from build123d import *

# Parameters (mm, degrees)
BOSS_EXTRUDE1_DEPTH = 34
BOSS_EXTRUDE4_START = -34
SKETCH2_R           = 1.35
BOSS_EXTRUDE4_DEPTH = 3
BOSS_EXTRUDE5_START = 3
SKETCH3_R           = 1.35
BOSS_EXTRUDE5_DEPTH = 3
CUT_EXTRUDE1_REACH  = 149.269
SKETCH4_W           = 50
SKETCH4_H           = 5
SKETCH4_H_2         = 10
CUT_EXTRUDE3_REACH  = 122.462
SKETCH5_W           = 5
SKETCH5_H           = 25


with BuildPart() as part:
    # Sketch1 → Boss-Extrude1 (new body)
    with BuildSketch(Plane.XY):
        Polygon((-115.55, 0), (0, 0), (0, 3), (-114.069788366, 3), (-136.169180916, 31.825294631), (-138.55, 30), align=None)
    extrude(amount=BOSS_EXTRUDE1_DEPTH)

    # Sketch2 → Boss-Extrude4 (add)
    # profile 1 of 3: a face of its own
    with BuildSketch(Plane.XY.offset(34).offset(BOSS_EXTRUDE4_START)):
        Polygon((0, 3), (-114.069788366, 3), (-136.169180916, 31.825294631), (-138.55, 30), (-115.55, 0), (0, 0), align=None)
    # profile 2 of 3: a face of its own
    with BuildSketch(Plane.XY.offset(34).offset(BOSS_EXTRUDE4_START)):
        Polygon((-34.075, 36.51210805), (-34.075, 3), (0, 3), (0, 8.6), (-28.475, 8.6), (-28.475, 36.51210805), align=None)
        with Locations((-25.975, 5.8)):
            Circle(SKETCH2_R, mode=Mode.SUBTRACT)
        with Locations((-3.975, 5.8)):
            Circle(SKETCH2_R, mode=Mode.SUBTRACT)
        with Locations((-31.275, 12.1)):
            Circle(SKETCH2_R, mode=Mode.SUBTRACT)
        with Locations((-31.275, 34.1)):
            Circle(SKETCH2_R, mode=Mode.SUBTRACT)
    # profile 3 of 3: a face of its own
    with BuildSketch(Plane.XY.offset(34).offset(BOSS_EXTRUDE4_START)):
        Polygon((-104.069788366, 3), (-114.069788366, 3), (-136.169180916, 31.825294631), (-138.55, 30), (-115.55, 0), (0, 0), (0, 3), (-34.075, 3), (-100.504119084, 3), align=None)
    extrude(amount=-BOSS_EXTRUDE4_DEPTH)

    # Sketch3 → Boss-Extrude5 (add)
    with BuildSketch(Plane.XY.offset(34).offset(BOSS_EXTRUDE5_START)):
        Polygon((0, 0), (0, 3), (0, 8.6), (-28.475, 8.6), (-28.475, 36.51210805), (-34.075, 36.51210805), (-34.075, 3), (-114.069788366, 3), (-136.169180916, 31.825294631), (-138.55, 30), (-115.55, 0), align=None)
        with Locations((-31.275, 34.1)):
            Circle(SKETCH3_R, mode=Mode.SUBTRACT)
        with Locations((-31.275, 12.1)):
            Circle(SKETCH3_R, mode=Mode.SUBTRACT)
        with Locations((-25.975, 5.8)):
            Circle(SKETCH3_R, mode=Mode.SUBTRACT)
        with Locations((-3.975, 5.8)):
            Circle(SKETCH3_R, mode=Mode.SUBTRACT)
    extrude(amount=-BOSS_EXTRUDE5_DEPTH)

    # Sketch4 → Cut-Extrude1 (cut, up to next)
    with BuildSketch(Plane(origin=(0, 3, 0), x_dir=(1, 0, 0), z_dir=(0, 1, 0)), mode=Mode.PRIVATE) as cut_extrude1_sk1:
        with Locations((-79.069788366, -4.5)):
            Rectangle(SKETCH4_W, SKETCH4_H)
    cut_extrude1_tool1 = extrude(cut_extrude1_sk1.sketch, amount=-CUT_EXTRUDE1_REACH, mode=Mode.PRIVATE) & part.part
    # Sketch4 → Cut-Extrude1 (cut, up to next)
    with BuildSketch(Plane(origin=(0, 3, 0), x_dir=(1, 0, 0), z_dir=(0, 1, 0)), mode=Mode.PRIVATE) as cut_extrude1_sk2:
        with Locations((-79.069788366, -29.5)):
            Rectangle(SKETCH4_W, SKETCH4_H)
    cut_extrude1_tool2 = extrude(cut_extrude1_sk2.sketch, amount=-CUT_EXTRUDE1_REACH, mode=Mode.PRIVATE) & part.part
    # Sketch4 → Cut-Extrude1 (cut, up to next)
    with BuildSketch(Plane(origin=(0, 3, 0), x_dir=(1, 0, 0), z_dir=(0, 1, 0)), mode=Mode.PRIVATE) as cut_extrude1_sk3:
        with Locations((-79.069788366, -17)):
            Rectangle(SKETCH4_W, SKETCH4_H_2)
    cut_extrude1_tool3 = extrude(cut_extrude1_sk3.sketch, amount=-CUT_EXTRUDE1_REACH, mode=Mode.PRIVATE) & part.part
    add(cut_extrude1_tool1.solids().sort_by_distance((-79.069788, 3, 4.5))[0], mode=Mode.SUBTRACT)
    add(cut_extrude1_tool2.solids().sort_by_distance((-79.069788, 3, 29.5))[0], mode=Mode.SUBTRACT)
    add(cut_extrude1_tool3.solids().sort_by_distance((-79.069788, 3, 17))[0], mode=Mode.SUBTRACT)

    # Sketch5 → Cut-Extrude3 (cut, up to next)
    with BuildSketch(Plane(origin=(-70.393848516, -53.968617195, 0), x_dir=(0, 0, -1), z_dir=(0.7936063612919156, 0.6084315436571361, 0)), mode=Mode.PRIVATE) as cut_extrude3_sk1:
        with Locations((-19.5, 90.606381212)):
            Rectangle(SKETCH5_W, SKETCH5_H)
    cut_extrude3_tool1 = extrude(cut_extrude3_sk1.sketch, amount=-CUT_EXTRUDE3_REACH, mode=Mode.PRIVATE) & part.part
    # Sketch5 → Cut-Extrude3 (cut, up to next)
    with BuildSketch(Plane(origin=(-70.393848516, -53.968617195, 0), x_dir=(0, 0, -1), z_dir=(0.7936063612919156, 0.6084315436571361, 0)), mode=Mode.PRIVATE) as cut_extrude3_sk2:
        with Locations((-14.5, 90.606381212)):
            Rectangle(SKETCH5_W, SKETCH5_H)
    cut_extrude3_tool2 = extrude(cut_extrude3_sk2.sketch, amount=-CUT_EXTRUDE3_REACH, mode=Mode.PRIVATE) & part.part
    # Sketch5 → Cut-Extrude3 (cut, up to next)
    with BuildSketch(Plane(origin=(-70.393848516, -53.968617195, 0), x_dir=(0, 0, -1), z_dir=(0.7936063612919156, 0.6084315436571361, 0)), mode=Mode.PRIVATE) as cut_extrude3_sk3:
        with Locations((-4.5, 90.606381212)):
            Rectangle(SKETCH5_W, SKETCH5_H)
    cut_extrude3_tool3 = extrude(cut_extrude3_sk3.sketch, amount=-CUT_EXTRUDE3_REACH, mode=Mode.PRIVATE) & part.part
    # Sketch5 → Cut-Extrude3 (cut, up to next)
    with BuildSketch(Plane(origin=(-70.393848516, -53.968617195, 0), x_dir=(0, 0, -1), z_dir=(0.7936063612919156, 0.6084315436571361, 0)), mode=Mode.PRIVATE) as cut_extrude3_sk4:
        with Locations((-29.5, 90.606381212)):
            Rectangle(SKETCH5_W, SKETCH5_H)
    cut_extrude3_tool4 = extrude(cut_extrude3_sk4.sketch, amount=-CUT_EXTRUDE3_REACH, mode=Mode.PRIVATE) & part.part
    add(cut_extrude3_tool1.solids().sort_by_distance((-125.521629, 17.937183, 19.5))[0], mode=Mode.SUBTRACT)
    add(cut_extrude3_tool2.solids().sort_by_distance((-125.521629, 17.937183, 14.5))[0], mode=Mode.SUBTRACT)
    add(cut_extrude3_tool3.solids().sort_by_distance((-125.521629, 17.937183, 4.5))[0], mode=Mode.SUBTRACT)
    add(cut_extrude3_tool4.solids().sort_by_distance((-125.521629, 17.937183, 29.5))[0], mode=Mode.SUBTRACT)


solid = part.part
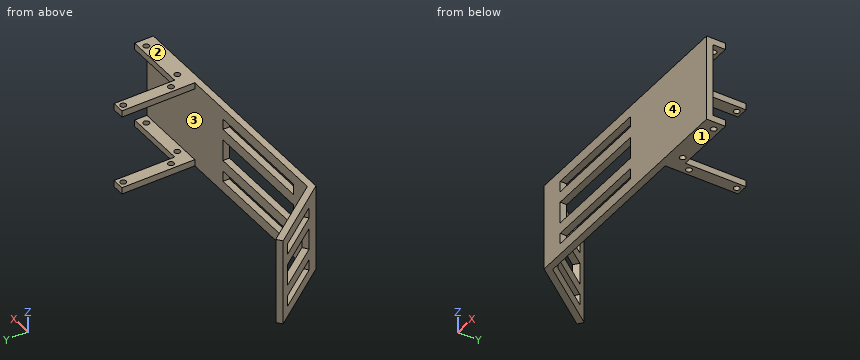
Read the model definition and answer for the solid it produces. Units are mm, in the model's axes. Face numbers are marked on the shaded views. Coordinates: 2 decimals unless noted, no trailing zeros. Loops run counter-clockwise (first coordinate to the right, second up) from the corner with the lowest first, then second, coordinate; pieces in that order, holes last. Notation, with made-up numbers: (-29.75, 49) -> (24.25, 49) arc R27 ccw to (24.25, 79) -> close; hole circle Ø9 at (14.5, 79). An arc over 180 degrees is marked (long way). Write item = value, one per line. Start each with the question number.
1) The part is cut by section D-D, the plane y = 12.1. State how many separate pieces and enclosed holes the cut face has, plus the area to 3 significant figures.
2) The mould has two halves that part along Z. Classify the marked faces 1, 2, 3 and 4: pulls with the +Z half, pulls with the -Z half, needs draft (parallel to the pull), parting line crosses it, or undercut.
3) The part is cut by section C-C, the plane x = -64.5. Determine the outline of the cut face in (y, z), plus the area to 3 significant figures.
4) The part is cut by section B-B, the plane z = 29. Determine the outline of the cut face in (x, y), plus the area to 3 significant figures.
5) Given P1, Ø1.5, axis at y = 27.5, z = 11.5, coming from the +X side; P2, Ø1.6, axis at x = -31.275, y = 12.1, coming from the +Z side; P3, Ø10, axis at y = 32.5, z = 9.5, coming from the +X side; P4, Ø2.5, axis at y = 17.5, z = -2, coming from the +X side (3 decimals), each flat-ended and moving along its own axis, determine where each tip first touches the part or whether it passes through.
6) Find the intervals of material crossed by L1, parallel to Z at x = -29, y = 34.5; L2, parallel to X at y = 7, z = 35 (3 decimals); L3, parallel to X at y = 12, z = 35 (3 decimals), in increasing order. Write a range as from..to.
7) The part is cut by section A-A, the plane y = 34.1. Determine the outline of the cut face in (x, z) (3 decimals).
Result:
q1.separate_pieces = 8
q1.enclosed_holes = 0
q1.area = 93.0 mm²
q2.face_1 = pulls with the -Z half
q2.face_2 = pulls with the +Z half
q2.face_3 = undercut
q2.face_4 = needs draft
q3.outline = (0, -3) -> (3, -3) -> (3, 2) -> (0, 2) -> close; (0, 7) -> (3, 7) -> (3, 12) -> (0, 12) -> close; (0, 22) -> (3, 22) -> (3, 27) -> (0, 27) -> close; (0, 32) -> (3, 32) -> (3, 37) -> (0, 37) -> close
q3.area = 60.0 mm²
q4.outline = (-138.55, 30) -> (-135.51, 26.03) -> (-133.13, 27.86) -> (-136.17, 31.83) -> close; (-120.3, 6.19) -> (-115.55, 0) -> (-104.07, 0) -> (-104.07, 3) -> (-114.07, 3) -> (-117.92, 8.02) -> close; (-54.07, 0) -> (0, 0) -> (0, 3) -> (-54.07, 3) -> close
q4.area = 231 mm²
q5.P1 = -132.28
q5.P2 = through
q5.P3 = -132.85
q5.P4 = -28.475
q6.L1 = -3..0, 34..37
q6.L2 = -120.917..-117.136, -34.075..-26.593, -25.357..-4.593, -3.357..0
q6.L3 = -124.75..-120.97, -34.075..-32.621, -29.929..-28.475
q7.outline = (-34.075, -3) -> (-32.625, -3) -> (-32.625, 0) -> (-34.075, 0) -> close; (-34.075, 34) -> (-32.625, 34) -> (-32.625, 37) -> (-34.075, 37) -> close; (-29.925, -3) -> (-28.475, -3) -> (-28.475, 0) -> (-29.925, 0) -> close; (-29.925, 34) -> (-28.475, 34) -> (-28.475, 37) -> (-29.925, 37) -> close
